from build123d import *

# Parameters (mm, degrees)
SKETCH1_R           = 1.5
BOSS_EXTRUDE1_DEPTH = 6
SKETCH2_W           = 28.99967905
SKETCH2_H           = 5.960844098
SKETCH2_W_2         = 10.731611964
CUT_EXTRUDE1_DEPTH  = 14


with BuildPart() as part:
    # Sketch1 → Boss-Extrude1 (new body)
    with BuildSketch(Plane(origin=(0, 0, 0), x_dir=(1, 0, 0), z_dir=(0, 1, 0))):
        with BuildLine():
            Line((0, 8), (122, 8))
            ThreePointArc((122, 8), (130, 0), (122, -8))
            Line((122, -8), (0, -8))
            ThreePointArc((0, -8), (-8, 0), (0, 8))
        make_face()
        Circle(SKETCH1_R, mode=Mode.SUBTRACT)
        with Locations((122, 0)):
            Circle(SKETCH1_R, mode=Mode.SUBTRACT)
    extrude(amount=BOSS_EXTRUDE1_DEPTH)

    # Sketch2 → Cut-Extrude1 (cut)
    with BuildSketch(Plane(origin=(0, 6, 0), x_dir=(1, 0, 0), z_dir=(0, 1, 0))):
        with Locations((30.5, 0)):
            Rectangle(SKETCH2_W, SKETCH2_H)
        with Locations((10.634354493, 0)):
            Rectangle(SKETCH2_W_2, SKETCH2_H)
        Polygon((105.999839525, 2.980422049), (77.000160475, 2.980422049), (77.000160475, -2.980422049), (105.999839525, -2.980422049), (116.731451489, -2.980422049), (116.731451489, 2.980422049), align=None)
    extrude(amount=-CUT_EXTRUDE1_DEPTH, mode=Mode.SUBTRACT)


solid = part.part
Model file for the job. Use its own axes, mm. A direction names the side the tool comes from. Give positions to 0.01 mm unless a question says otherwise; leave off trailing zeros. Write each loop counter-clockwise with the first axis right and the second up, starting at its lowest first coordinate (ties: lowest second). Pieces come first, ordered by that corner, then holes. Notation, with made-up numbers: M 31.5,-33.75 L 73.5,-33.75 A28 cw 73.5,-12.75 Z; hole C -32.5,55 d2. An arc over 180 degrees is marked long. One line per item, written item: value. Start each with the question number.
Q1. Saw through at C-C, the plane z = 0. Write the cut outline in (x, y), plus the area to 3 significant figures.
Q2. Saw through at A-A, the plane x = 104. Write the cut outline in (y, z).
Q3. 3-axis set-ups, long thin cutter, end or side, ignore diameter. For faces 4 (the flat face through (116.731, 3, 0)), 5 (the cylindrical face through (130, 3, 0)): which of +Z, -Z, +X, -X, +Y, -Y reach the whole face in a straight line?
Q4. Saw through at B-B, the plane y = 5.1. Write the cut outline in (x, z).
Q5. Two-plate mould, pull along Z, no slides. Class faces 1 (the flat face through (25, 3, -2.98)), 2 (the flat face through (62, 3, 8)), 3 (the cylindrical face through (-8, 3, 0)): +Z half, -Z half, draft (parallel to the pull), parting line (faces both ways), or undercut.
Q6. Drop flat-ended pins along their axis: pin 1 Ø1.5 at (y, z) = (4.5, 3.5) entering from +X; pin 2 Ø5 at (x, z) = (122, 0) entering from +Y; pin 3 Ø1.8 at (x, z) = (0, 0) entering from +Y; pin 4 Ø1.8 at (y, z) = (3, -1.5) entering from -X. Give the stop position or say it passes through.
Q7. Probe probe 1 along X at (y, z) = (3.25, 0); probe 2 along Z at (x, y) = (17, 1.2); probe 3 along X at (y, z) = (2.55, 2.5). List the from-to ranges inside material, lowest first. Write a range as [from, to].
Output values:
1. outline: M -8,0 L -1.5,0 L -1.5,6 L -8,6 Z; M 1.5,0 L 5.27,0 L 5.27,6 L 1.5,6 Z; M 45,0 L 77,0 L 77,6 L 45,6 Z; M 116.73,0 L 120.5,0 L 120.5,6 L 116.73,6 Z; M 123.5,0 L 130,0 L 130,6 L 123.5,6 Z
1. area: 315 mm²
2. outline: M 0,-8 L 6,-8 L 6,-2.98 L 0,-2.98 Z; M 0,2.98 L 6,2.98 L 6,8 L 0,8 Z
3. face 4: +Y, -Y
3. face 5: +X, +Y, -Y
4. outline: M 0,-8 L 122,-8 A8 ccw 122,8 L 0,8 A8 ccw Z; hole C 0,0 d3; hole M 5.27,-2.98 L 45,-2.98 L 45,2.98 L 5.27,2.98 Z; hole M 77,-2.98 L 116.73,-2.98 L 116.73,2.98 L 77,2.98 Z; hole C 122,0 d3
5. face 1: undercut
5. face 2: +Z half
5. face 3: parting line
6. pin 1: stops at x = 129.51
6. pin 2: stops at y = 6
6. pin 3: passes through
6. pin 4: stops at x = -7.98
7. probe 1: x = [-8, -1.5], [1.5, 5.27], [45, 77], [116.73, 120.5], [123.5, 130]
7. probe 2: z = [-8, -2.98], [2.98, 8]
7. probe 3: x = [-7.6, 5.27], [45, 77], [116.73, 129.6]
